For this review, take the finished solid that the model builds, in its own axes (mm). A direction names the side the tool comes from. Coordinates: 2 decimals unless noted, no trailing zeros. Write each loop counter-clockwise with the first axis right and the second up, starting at its lowest first coordinate (ties: lowest second). Pieces come first, ordered by that corner, then holes. Notation, with made-up numbers: (22, 66.25) -> (27, 66.25) arc R17 ccw to (27, 94.25) -> close; hole circle Ø8 at (82.5, 66.5). An arc over 180 degrees is marked (long way). Put each result on its own line as item: value. Start each with the question number.
Item 1: Consider section C-C on x = 1.5. Give the boundary of the cut face in (y, z).
Item 2: The part is to be moulded in two halves that separate along Z. For faces 4 (the cylindrical face through (-27.22, -4.049, -28.073)), 5 (the cylindrical face through (-26.052, -4.965, 15.803)), 6 (the flat face through (10, -10, 26.936)), 7 (the flat face through (10, 0, -5)), say which applies: +Z half, -Z half, draft (parallel to the pull), parting line (faces both ways), or undercut.
Item 3: Consider section D-D on y = -9.5. Give the boundary of the cut face in (x, z).
Item 4: Consider section B-B on y = -4.5. Give the number of separate pieces and of enclosed holes in the cut face, and give its area (3 significant figures).
Item 5: Consider section A-A on z = -33. Give the boundary of the cut face in (x, y).
Item 6: To check wall thickness, follow L1, parallel to Z at x = -27, y = -6.25; L2, parallel to Z at x = 50.5, y = -10.5; L3, parallel to X at y = -12.25, z = -22.5. State the ranges of each line that lie inside material, in increasing order.
Item 7: For faces 1 (the flat face through (-41.661, -12, -6)), 2 (the flat face through (10, -14, -35.564)), 3 (the flat face through (-40, -22, 7.936)), list the 3-axis set-ups (+Z, -Z, +X, -X, +Y, -Y) from which the entire face can be reached by the end or side of a thin tool; tool diameter is ignored.
Item 8: Insertion check: P1, Ø5.5, axis at x = -27, z = -28.5, coming from the -Y side; P2, Ø1, axis at x = 21, y = -21.5, coming from the +Z side; P3, Ø5, axis at x = -19.5, z = 13.5, coming from the -Y side. Each pin has a flat end and moves straight along its axis. Give the tip position at first contact, or say it passes through.
```python
from build123d import *

# Parameters (mm, degrees)
F0_W      = 105
F0_H      = 65
F1_DEPTH  = 25
F3_DEPTH  = 22.5
F4_W      = 5
F4_H      = 19
F5_DEPTH  = 2.5
F6_W      = 5
F6_H      = 19
F7_DEPTH  = 2.5
F9_DEPTH  = 2.5
F10_R     = 2.403973
F11_DEPTH = 5
F12_R     = 0.874474
F12_R_2   = 0.999999
F12_R_3   = 0.846332
F12_R_4   = 1
F13_DEPTH = 7


with BuildPart() as f1:
    # F0 (on Front) → F1 (new body)
    with BuildSketch(Plane.XZ):
        with Locations((10.83879, -5.564056)):
            Rectangle(F0_W, F0_H)
    extrude(amount=F1_DEPTH)

    # F2 (on face) → F3 (cut)
    with BuildSketch(Plane.XZ.offset(25)):
        Polygon((12.475623, 24.435944), (-39.16121, 24.435944), (-39.16121, -11.767991), (-39.16121, -35.564056), (11.927005, -35.564056), (60.83879, -35.564056), (60.83879, -26.717814), (60.83879, 24.435944), align=None)
    extrude(amount=-F3_DEPTH, mode=Mode.SUBTRACT)

    # F4 (on face) → F5 (cut)
    with BuildSketch(Plane(origin=(-41.66121, 0, 0), x_dir=(0, -1, 0), z_dir=(-1, 0, 0))):
        with Locations((22.5, 17.435944)):
            Rectangle(F4_W, F4_H)
    extrude(amount=-F5_DEPTH, mode=Mode.SUBTRACT)

    # F6 (on face) → F7 (cut)
    with BuildSketch(Plane.YZ.offset(63.33879)):
        with Locations((-22.5, 17.435944)):
            Rectangle(F6_W, F6_H)
    extrude(amount=-F7_DEPTH, mode=Mode.SUBTRACT)

    # F8 (on face) → F9 (cut)
    with BuildSketch(Plane.XY.offset(26.935944)):
        Polygon((-39.16121, -20), (-39.16121, -22.5), (-39.16121, -25), (60.83879, -25), (60.83879, -20), align=None)
    extrude(amount=-F9_DEPTH, mode=Mode.SUBTRACT)

    # F10 (on face) → F11 (join)
    with BuildSketch(Plane.XZ.offset(2.5)):
        with Locations((48.83879, 17.935944)):
            Circle(F10_R)
        with Locations((-27.16121, -29.064056)):
            Circle(F10_R)
        with Locations((48.83879, -29.064056)):
            Circle(F10_R)
        with Locations((-27.16121, 17.935944)):
            Circle(F10_R)
    extrude(amount=F11_DEPTH)

    # F12 (on face) → F13 (cut)
    with BuildSketch(Plane.XZ.offset(7.5)):
        with Locations((48.756924, 17.979905)):
            Circle(F12_R)
        with Locations((48.756924, -29.064033)):
            Circle(F12_R_2)
        with Locations((-27.16121, 17.935944)):
            Circle(F12_R_3)
        with Locations((-27.089426, -29.064033)):
            Circle(F12_R_4)
    extrude(amount=-F13_DEPTH, mode=Mode.SUBTRACT)


solid = f1.part
```
Return value:
1. outline: (-25, -38.06) -> (0, -38.06) -> (0, 26.94) -> (-20, 26.94) -> (-20, 24.44) -> (-2.5, 24.44) -> (-2.5, -35.56) -> (-25, -35.56) -> close
2. face 4: undercut
2. face 5: undercut
2. face 6: +Z half
2. face 7: draft
3. outline: (-41.66, -38.06) -> (63.34, -38.06) -> (63.34, 26.94) -> (-41.66, 26.94) -> close; hole (-39.16, -35.56) -> (60.84, -35.56) -> (60.84, 24.44) -> (-39.16, 24.44) -> close
4. separate pieces: 5
4. enclosed holes: 5
4. area: 887 mm^2
5. outline: (-41.66, -25) -> (-39.16, -25) -> (-39.16, -2.5) -> (60.84, -2.5) -> (60.84, -25) -> (63.34, -25) -> (63.34, 0) -> (-41.66, 0) -> close
6. L1: -38.06 to -35.56, -31.46 to -30.06, -28.07 to -26.67, 15.54 to 17.11, 18.77 to 20.33, 24.44 to 26.94
6. L2: -38.06 to -35.56, 24.44 to 26.94
6. L3: -41.66 to -39.16, 60.84 to 63.34
7. face 1: +Z, -Z, -X, +Y, -Y
7. face 2: -Y
7. face 3: +Z, +X, -X, -Y
8. P1: y = -7.5
8. P2: z = -35.56
8. P3: y = -2.5
